Could you check a few things on this model? Use its own coordinates, in mm. Face numbers are marked on the shaded views. A direction names the side the tool comes from. Coordinates: 2 decimals unless noted, no trailing zeros. Loops run counter-clockwise (first coordinate to the right, second up) from the corner with the lowest first, then second, coordinate; pieces in that order, holes last. Notation, with made-up numbers: (44, -17.75) -> (53, -17.75) arc R19 cw to (53, 6.25) -> close; hole circle Ø2 at (-15, -8). An arc over 180 degrees is marked (long way). One line per question, with ' | ' between items. Start each with the question number.
(1) Suppose I cut it at D-D (z = 13.75). Give the number of separate pieces and of enclosed holes in the cut face, plus the area to 3 significant figures.
(2) Suppose I cut it at A-A (y = 10.5). Please give me the cut outline in (x, z) (1 decimal), plus the area to 3 significant figures.
(3) Suppose I cut it at C-C (z = 6.75). Please give me the cut outline in (x, y) (1 decimal), plus the area to 3 significant figures.
(4) I'm going to push flat-ended pins straight in: pin 1 Ø1.7 at (x, y) = (55, -10) entering from +Z; pin 2 Ø3.5 at (x, y) = (-38.5, -24) entering from +Z; pin 3 Ø2 at (x, y) = (28, 13.5) entering from +Z; pin 4 Ø1.4 at (x, y) = (53.18, -29.15) entering from -Z. Where does each tip first touch, or does it pass through?
(5) If we mould it in two halves opening along X, with no side actions, what happens to the marked faces 1, 2 and 3? For each: pulls with the +X half, pulls with the -X half, needs draft (parallel to the pull), parting line crosses it, or undercut.
(6) If I drill on line 1 along Y through (x, z) = (-45.8, 2.35); line 2 along Y through (x, z) = (-24.5, 13.5); line 3 along X through (y, z) = (2.5, 13) (1 decimal), over which ranges is the centre line in solid material (lowest first)?
(7) Suppose I cut it at B-B (x = -42). Please give me the cut outline in (y, z).
(8) Which directions (+Z, -Z, +X, -X, +Y, -Y) give clear straight access to the entire face, cutting with the end or side of a thin tool? Please do the marked faces 4 and 5.
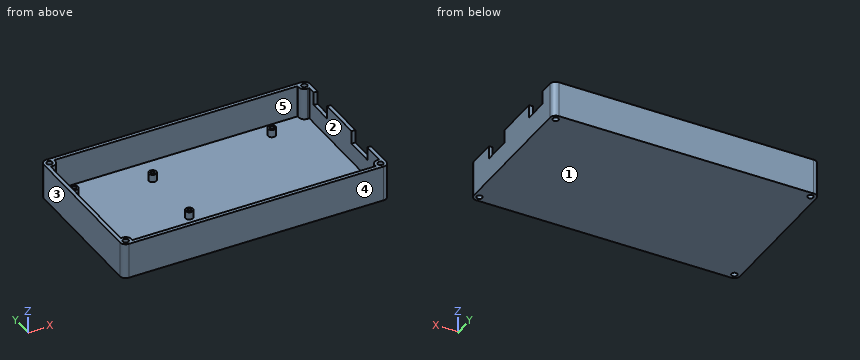
```python
from build123d import *

# Parameters (mm, degrees)
F1_W      = 111.125
F1_H      = 63.0682
F2_DEPTH  = 1.5875
F3_W      = 111.125
F3_H      = 63.0682
F3_R      = 1.190625
F4_DEPTH  = 13.335
F5_R      = 2.38125
F6_W      = 12.065
F6_H      = 5.5245
F6_W_2    = 10.287
F7_DEPTH  = 1.5875
F8_R      = 1.5875
F8_R_2    = 0.79375
F9_DEPTH  = 3.175
F10_R     = 1.190625
F11_DEPTH = 14.9235


with BuildPart() as f2:
    # F1 (on Top) → F2 (new body)
    with BuildSketch(Plane.XY):
        Rectangle(F1_W, F1_H)
    extrude(amount=F2_DEPTH)

    # F3 (on face) → F4 (join)
    with BuildSketch(Plane.XY.offset(1.5875)):
        Rectangle(F3_W, F3_H)
        with Locations((-53.18125, -29.15285)):
            Circle(F3_R, mode=Mode.SUBTRACT)
        with Locations((53.18125, -29.15285)):
            Circle(F3_R, mode=Mode.SUBTRACT)
        with BuildLine():
            Line((53.18125, 26.7716), (53.975, 26.7716))
            Line((53.975, 26.7716), (53.975, -26.7716))
            Line((53.975, -26.7716), (53.18125, -26.7716))
            ThreePointArc((53.18125, -26.7716), (51.497452, -27.469052), (50.8, -29.15285))
            Line((50.8, -29.15285), (50.8, -29.9466))
            Line((50.8, -29.9466), (-50.8, -29.9466))
            Line((-50.8, -29.9466), (-50.8, -29.15285))
            ThreePointArc((-50.8, -29.15285), (-51.497452, -27.469052), (-53.18125, -26.7716))
            Line((-53.18125, -26.7716), (-53.975, -26.7716))
            Line((-53.975, -26.7716), (-53.975, 26.7716))
            Line((-53.975, 26.7716), (-53.18125, 26.7716))
            ThreePointArc((-53.18125, 26.7716), (-51.497452, 27.469052), (-50.8, 29.15285))
            Line((-50.8, 29.15285), (-50.8, 29.9466))
            Line((-50.8, 29.9466), (50.8, 29.9466))
            Line((50.8, 29.9466), (50.8, 29.15285))
            ThreePointArc((50.8, 29.15285), (51.497452, 27.469052), (53.18125, 26.7716))
        make_face(mode=Mode.SUBTRACT)
        with Locations((-53.18125, 29.15285)):
            Circle(F3_R, mode=Mode.SUBTRACT)
        with Locations((53.18125, 29.15285)):
            Circle(F3_R, mode=Mode.SUBTRACT)
    extrude(amount=F4_DEPTH)

    # F5
    f5_edges = [f2.edges().sort_by_distance(p)[0] for p in [
        (55.5625, -31.5341, 7.46125),
        (55.5625, 31.5341, 7.46125),
        (-55.5625, -31.5341, 7.46125),
        (-55.5625, 31.5341, 7.46125),
    ]]
    fillet(f5_edges, radius=F5_R)

    # F6 (on face) → F7 (cut, through all)
    with BuildSketch(Plane.YZ.offset(55.5625)):
        with Locations((-11.557, 12.16025)):
            Rectangle(F6_W, F6_H)
        with Locations((18.288, 12.16025)):
            Rectangle(F6_W_2, F6_H)
    extrude(amount=-F7_DEPTH, mode=Mode.SUBTRACT)

    # F8 (on face) → F9 (join)
    with BuildSketch(Plane.XY.offset(1.5875)):
        with Locations((-45.8, 23.7716)):
            Circle(F8_R)
        with Locations((-45.8, 23.7716)):
            Circle(F8_R_2, mode=Mode.SUBTRACT)
        with Locations((-39.3, -24.2284)):
            Circle(F8_R)
        with Locations((-39.3, -24.2284)):
            Circle(F8_R_2, mode=Mode.SUBTRACT)
        with Locations((-15.8, 18.7716)):
            Circle(F8_R)
        with Locations((-15.8, 18.7716)):
            Circle(F8_R_2, mode=Mode.SUBTRACT)
        with Locations((-15.8, -9.2284)):
            Circle(F8_R)
        with Locations((-15.8, -9.2284)):
            Circle(F8_R_2, mode=Mode.SUBTRACT)
        with Locations((36.7, 23.7716)):
            Circle(F8_R)
        with Locations((36.7, 23.7716)):
            Circle(F8_R_2, mode=Mode.SUBTRACT)
        with Locations((36.7, -24.2284)):
            Circle(F8_R)
        with Locations((36.7, -24.2284)):
            Circle(F8_R_2, mode=Mode.SUBTRACT)
    extrude(amount=F9_DEPTH)

    # F10 (on face) → F11 (cut, through all)
    with BuildSketch(Plane.XY.offset(14.9225)):
        with Locations((-53.18125, 29.15285)):
            Circle(F10_R)
        with Locations((-53.18125, -29.15285)):
            Circle(F10_R)
        with Locations((53.18125, -29.15285)):
            Circle(F10_R)
        with Locations((53.18125, 29.15285)):
            Circle(F10_R)
    extrude(amount=-F11_DEPTH, mode=Mode.SUBTRACT)


solid = f2.part
```
Checks:
1) separate pieces: 2 | enclosed holes: 4 | area: 520 mm^2
2) outline: (-55.6, 0) -> (55.6, 0) -> (55.6, 14.9) -> (54, 14.9) -> (54, 1.6) -> (-54, 1.6) -> (-54, 14.9) -> (-55.6, 14.9) -> close | area: 219 mm^2
3) outline: (-55.6, -29.2) arc R2.4 ccw to (-53.2, -31.5) -> (53.2, -31.5) arc R2.4 ccw to (55.6, -29.2) -> (55.6, 29.2) arc R2.4 ccw to (53.2, 31.5) -> (-53.2, 31.5) arc R2.4 ccw to (-55.6, 29.2) -> close; hole circle Ø2.4 at (-53.2, -29.2); hole circle Ø2.4 at (-53.2, 29.2); hole (-54, -26.8) -> (-53.2, -26.8) arc R2.4 cw to (-50.8, -29.2) -> (-50.8, -29.9) -> (50.8, -29.9) -> (50.8, -29.2) arc R2.4 cw to (53.2, -26.8) -> (54, -26.8) -> (54, 26.8) -> (53.2, 26.8) arc R2.4 cw to (50.8, 29.2) -> (50.8, 29.9) -> (-50.8, 29.9) -> (-50.8, 29.2) arc R2.4 cw to (-53.2, 26.8) -> (-54, 26.8) -> close; hole circle Ø2.4 at (53.2, -29.2); hole circle Ø2.4 at (53.2, 29.2) | area: 556 mm^2
4) pin 1: stops at z = 9.4 | pin 2: stops at z = 4.76 | pin 3: stops at z = 1.59 | pin 4: passes through
5) face 1: needs draft | face 2: undercut | face 3: pulls with the -X half
6) line 1: y = -31.53 to -29.95, 22.18 to 22.98, 24.57 to 25.36, 29.95 to 31.53 | line 2: y = -31.53 to -29.95, 29.95 to 31.53 | line 3: x = -55.6 to -54, 54 to 55.6
7) outline: (-31.53, 0) -> (31.53, 0) -> (31.53, 14.92) -> (29.95, 14.92) -> (29.95, 1.59) -> (-29.95, 1.59) -> (-29.95, 14.92) -> (-31.53, 14.92) -> close
8) face 4: +Z, -Z, +X, -X, -Y | face 5: +Z
